Check sheet for the modelled part. Datum: model origin and axes. Units: mm. Face numbers are marked on the shaded views. A direction names the side the tool comes from. Round coordinates to 2 decimals unless told otherwise and drop trailing zeros. Write each loop counter-clockwise with the first axis right and the second up, starting at its lowest first coordinate (ties: lowest second). Pieces come first, ordered by that corner, then holes. Notation, with made-up numbers: (52.5, -2.75) -> (101.5, -2.75) arc R30 cw to (101.5, 21.25) -> close; hole circle Ø6 at (71, 14.25). An arc over 180 degrees is marked (long way). One line per item, written item: value.
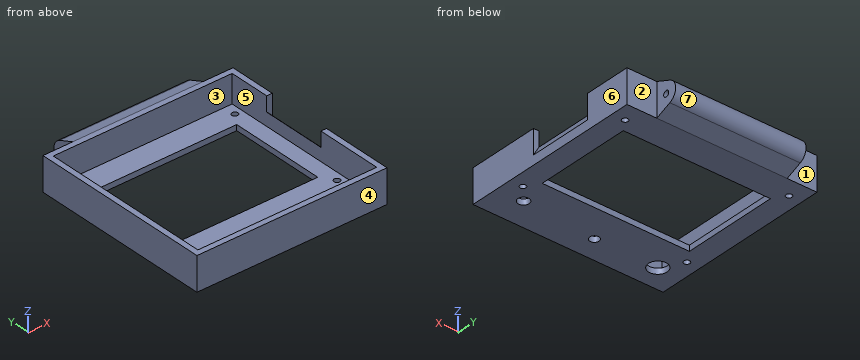
from build123d import *

# Parameters (mm, degrees)
ESBO_O2_W                = 18
ESBO_O2_H                = 98
RESSALTO_EXTRUS_O1_DEPTH = 51
CASCA1_T                 = -3
ESBO_O4_R                = 1.6
ESBO_O4_R_2              = 5
ESBO_O4_R_3              = 3
ESBO_O4_R_4              = 2.5
ESBO_O4_W                = 79
ESBO_O4_H                = 51.6
CORTE_EXTRUS_O1_DEPTH    = 3
ESBO_O5_R                = 1.6
RESSALTO_EXTRUS_O2_DEPTH = 102
ESBO_O6_W                = 16
ESBO_O6_H                = 12
CORTE_EXTRUS_O2_DEPTH    = 19
ESBO_O7_W                = 8
ESBO_O7_H                = 34.5
CORTE_EXTRUS_O3_DEPTH    = 10
CHANFRO1_SIZE            = 5
CHANFRO1_SIZE2           = 2.886751346


with BuildPart() as part:
    # Esboço2 → Ressalto-extrusão1 (new body, symmetric)
    with BuildSketch(Plane(origin=(0, 0, 0), x_dir=(0, 0, -1), z_dir=(1, 0, 0))):
        with Locations((9, 49)):
            Rectangle(ESBO_O2_W, ESBO_O2_H)
    extrude(amount=RESSALTO_EXTRUS_O1_DEPTH, both=True)

    # Casca1
    casca1_openings = [part.faces().sort_by_distance(p)[0] for p in [
        (0, 49, 0),
    ]]
    offset(amount=CASCA1_T, openings=casca1_openings, kind=Kind.INTERSECTION)

    # Esboço4 → Corte-extrusão1 (cut)
    with BuildSketch(Plane(origin=(0, 0, -18), x_dir=(1, 0, 0), z_dir=(0, 0, -1))):
        with Locations((-44, -23.5)):
            Circle(ESBO_O4_R)
        with Locations((-44, -88.5)):
            Circle(ESBO_O4_R)
        with Locations((44, -88.5)):
            Circle(ESBO_O4_R)
        with Locations((44, -23.5)):
            Circle(ESBO_O4_R)
        with Locations((-37.5, -12.7)):
            Circle(ESBO_O4_R_2)
        with Locations((36.75, -15.3)):
            Circle(ESBO_O4_R_3)
        with Locations((-3.8, -12.3)):
            Circle(ESBO_O4_R_4)
        with Locations((0, -56.2)):
            Rectangle(ESBO_O4_W, ESBO_O4_H)
    extrude(amount=-CORTE_EXTRUS_O1_DEPTH, mode=Mode.SUBTRACT)

    # Esboço5 → Ressalto-extrusão2 (add, through all)
    with BuildSketch(Plane(origin=(51, 0, 0), x_dir=(0, 0, -1), z_dir=(1, 0, 0))):
        with BuildLine():
            Line((14.538461538, 106.307692308), (18, 98))
            Line((18, 98), (0, 98))
            Line((0, 98), (3.461538462, 106.307692308))
            ThreePointArc((3.461538462, 106.307692308), (9, 110), (14.538461538, 106.307692308))
        make_face()
        with Locations((9, 104)):
            Circle(ESBO_O5_R, mode=Mode.SUBTRACT)
    extrude(amount=-RESSALTO_EXTRUS_O2_DEPTH)

    # Esboço6 → Corte-extrusão2 (cut, through all)
    with BuildSketch(Plane(origin=(0, 0, -18), x_dir=(-1, 0, 0), z_dir=(0, 0, -1))):
        with Locations((-43, 104)):
            Rectangle(ESBO_O6_W, ESBO_O6_H)
        with Locations((43, 104)):
            Rectangle(ESBO_O6_W, ESBO_O6_H)
    extrude(amount=-CORTE_EXTRUS_O2_DEPTH, mode=Mode.SUBTRACT)

    # Esboço7 → Corte-extrusão3 (cut)
    with BuildSketch(Plane(origin=(51, 0, 0), x_dir=(0, 0, -1), z_dir=(1, 0, 0))):
        with Locations((4, 55.75)):
            Rectangle(ESBO_O7_W, ESBO_O7_H)
    extrude(amount=-CORTE_EXTRUS_O3_DEPTH, mode=Mode.SUBTRACT)

    # Chanfro1
    chanfro1_edges = [part.edges().sort_by_distance(p)[0] for p in [
        (51, 55.75, -8),
    ]]
    chanfro1_side = [part.faces().sort_by_distance(p)[0] for p in [
        (51, 47.747983871, -9.927419355),
    ]]
    chamfer(chanfro1_edges, length=CHANFRO1_SIZE, length2=CHANFRO1_SIZE2, reference=chanfro1_side[0])


solid = part.part
Item 1: Sectioned sample at C-C (y = 23.5). Enter the section's corners in (x, z).
Result set:
outline: (-51, -18) -> (-45.6, -18) -> (-45.6, -15) -> (-48, -15) -> (-48, 0) -> (-51, 0) -> close; (-42.4, -18) -> (42.4, -18) -> (42.4, -15) -> (-42.4, -15) -> close; (45.6, -18) -> (51, -18) -> (51, 0) -> (48, 0) -> (48, -15) -> (45.6, -15) -> close
Item 2: Material ranges on line 1 along Y through (x, z) = (-44, -16.5); line 2 along Y through (x, z) = (-37.5, -17.1); line 3 along X through (y, z) = (23.5, -16.35), recorded low to high.
Result set:
line 1: 0 to 21.9, 25.1 to 86.9, 90.1 to 98
line 2: 0 to 7.7, 17.7 to 30.4, 82 to 98
line 3: -51 to -45.6, -42.4 to 42.4, 45.6 to 51
Item 3: Sectioned sample at D-D (x = 36.75). Enter the section's corners in (y, z), then the cut area to 3 significant figures.
Result set:
outline: (0, -18) -> (12.3, -18) -> (12.3, -15) -> (3, -15) -> (3, 0) -> (0, 0) -> close; (18.3, -18) -> (30.4, -18) -> (30.4, -15) -> (18.3, -15) -> close; (82, -18) -> (98, -18) -> (98, 0) -> (95, 0) -> (95, -15) -> (82, -15) -> close
area: 211 mm^2
Item 4: Sectioned sample at A-A (x = -18). Enter the section's corners in (y, z), then the cut area to 3 significant figures.
Result set:
outline: (0, -18) -> (30.4, -18) -> (30.4, -15) -> (3, -15) -> (3, 0) -> (0, 0) -> close; (82, -18) -> (98, -18) -> (106.31, -14.54) arc R6 ccw to (106.31, -3.46) -> (98, 0) -> (95, 0) -> (95, -15) -> (82, -15) -> close; hole circle Ø3.2 at (104, -9)
area: 371 mm^2
Item 5: Release check for a two-part mould opening along X. For the marked faces 5, 6 and 7 record: pulls with the +X half, pulls with the -X half, needs draft (parallel to the pull), parting line crosses it, or undercut.
Result set:
face 5: undercut
face 6: pulls with the +X half
face 7: needs draft
Item 6: Sectioned sample at B-B (y = 63). Enter the section's corners in (x, z).
Result set:
outline: (-51, -18) -> (-39.5, -18) -> (-39.5, -15) -> (-48, -15) -> (-48, 0) -> (-51, 0) -> close; (39.5, -18) -> (51, -18) -> (51, -13) -> (48.11, -8) -> (48, -8) -> (48, -15) -> (39.5, -15) -> close
Item 7: Tool access check on the marked faces 1, 2, 3 and 4. Record the directions out of +Z, -Z, +X, -X, +Y, -Y that give a thin tool (end or side, any length) a straight path to the whole face; none if there is none.
Result set:
face 1: +Z, -Z, -X, +Y
face 2: +Z, -Z, +X, +Y
face 3: +Z
face 4: +Z, -Z, +X, -X, -Y
Item 8: Depth check by flat-ended pin: pin 1 (2 mm diameter, centred on x = -37, z = -15.5, fed in from +Y); pin 2 (3.5 mm diameter, centred on y = 104, z = -9, fed in from +X); pin 3 (5 mm diameter, centred on x = 3.5, z = -3, fed in from +Y). Enter the tip coordinate at first touch or a pass-through.
Result set:
pin 1: y = 98
pin 2: x = 35
pin 3: y = 108.87
